Can you work these out from the model? Positions are in its coordinate system, mm. Face numbers are marked on the shaded views. A direction names the side the tool comes from. Give positions to 0.01 mm unless a question says otherwise; leave off trailing zeros. Loops run counter-clockwise (first coordinate to the right, second up) from the corner with the lowest first, then second, coordinate; pieces in that order, holes last. Notation, with made-up numbers: M 55,0 L 64,0 A12 ccw 64,12 Z; hole C -3,29 d11. An arc over 180 degrees is marked long. Answer as a JSON object with one key per item and string values.
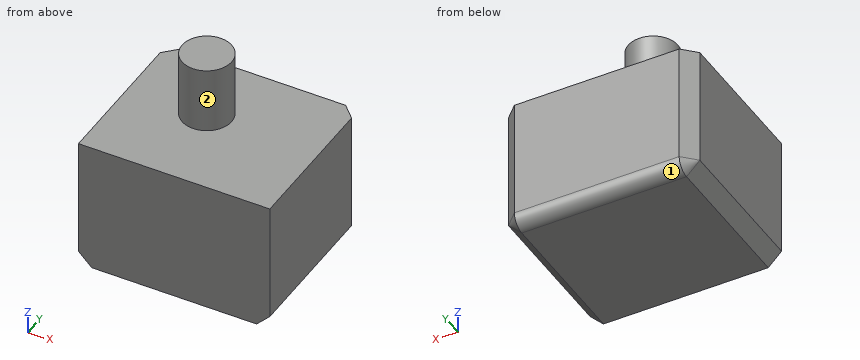
```python
from build123d import *

# Parameters (mm, degrees)
F0_W     = 36.594145
F0_H     = 61.4954829216
F1_DEPTH = 25.4
F2_DEPTH = 25.4
F3_R     = 5.08
F4_SIZE  = 5.07999
F5_R     = 9.4762574088
F6_DEPTH = 25.4


# Not quite as in the source:
# - a fillet or chamfer is up to 0.001 mm smaller than in the source, because OpenCascade refuses the exact size


with BuildPart() as f1:
    # F0 (on Top) → F1 (new body)
    with BuildSketch(Plane.XY):
        with Locations((-12.8837414086, -3.4645497799)):
            Rectangle(F0_W, F0_H)
        with Locations((23.7104035914, -3.4645497799)):
            Rectangle(F0_W, F0_H)
    extrude(amount=F1_DEPTH)

    # F2 (add): a face of the model
    f2_faces = [f1.faces().sort_by_distance(p)[0] for p in [
        (5.4133310914, -3.4645497799, 25.4),
    ]]
    extrude(f2_faces, amount=F2_DEPTH)

    # F3
    f3_edges = [f1.edges().sort_by_distance(p)[0] for p in [
        (5.413331, 27.283192, 0),
    ]]
    fillet(f3_edges, radius=F3_R)

    # F4 (size 5.08 in the source; OpenCascade refuses exactly that, so slightly less here)
    f4_edges = [f1.edges().sort_by_distance(p)[0] for p in [
        (-31.180814, 27.283192, 27.94),
        (42.007476, 27.283192, 27.94),
        (42.007476, -6.00455, 0),
    ]]
    chamfer(f4_edges, length=F4_SIZE)

    # F5 (on face) → F6 (join)
    with BuildSketch(Plane.XY.offset(50.8)):
        with Locations((-1.593567431, 1.0238895973)):
            Circle(F5_R)
    extrude(amount=F6_DEPTH)


solid = f1.part
```
1) Please list where these lines run through material, in increasing order: line 1 along Z through (x, y) = (11, 2.5); line 2 along Y through (x, z) = (2, 66); line 3 along Y through (x, z) = (4, 73). Write a range as from..to.
Answer list:
{"line 1": "0..50.8", "line 2": "-7.74..9.79", "line 3": "-6.63..8.67"}
2) Suppose I cut it at D-D, the plane z = 57.5. Write out the boundary of the cut face in (x, y).
Answer list:
{"outline": "C -1.59,1.02 d18.95"}
3) Suppose I cut it at A-A, the plane y = -1. Write out the boundary of the cut face in (x, z), and give its area (3 significant figures).
Answer list:
{"outline": "M -31.18,5.08 L -26.1,0 L 36.93,0 L 42.01,5.08 L 42.01,50.8 L 7.66,50.8 L 7.66,76.2 L -10.85,76.2 L -10.85,50.8 L -31.18,50.8 Z", "area": "4,160 mm^2"}
4) For the marked faces 1 and 2, which set-ups out of +Z, -Z, +X, -X, +Y, -Y let a thin tool reach every point of the face, with its end or its side?
Answer list:
{"face 1": "-Z, +X, -X, +Y", "face 2": "+Z"}
5) Will this pin go through, and if not, where does the flat tip stop? pin 1 Ø2 at (x, y) = (28.5, -24.5) entering from +Z.
Answer list:
{"pin 1": "z = 50.8"}
6) Suppose I cut it at B-B, the plane x = 34. Write out the boundary of the cut face in (y, z).
Answer list:
{"outline": "M -34.21,0 L 22.2,0 A5.08 ccw 27.28,5.08 L 27.28,50.8 L -34.21,50.8 Z"}
7) Suppose I cut it at C-C, the plane y = 19.5. Write out the boundary of the cut face in (x, z), and give its area (3 significant figures).
Answer list:
{"outline": "M -31.18,5.08 L -26.1,0 L 36.93,0 L 42.01,5.08 L 42.01,50.8 L -31.18,50.8 Z", "area": "3,690 mm^2"}
